from build123d import *

# Parameters (mm, degrees)
SKETCH1_W           = 150
SKETCH1_H           = 150
BOSS_EXTRUDE1_DEPTH = 3
SKETCH2_W           = 146
SKETCH2_H           = 146
BOSS_EXTRUDE2_DEPTH = 3
SKETCH3_W           = 142
SKETCH3_H           = 142
CUT_EXTRUDE1_DEPTH  = 3
EXTRUDE_THIN1_DEPTH = 3
CUT_EXTRUDE5_START  = -3
SKETCH5_W           = 71.2
SKETCH5_H           = 24.1
CUT_EXTRUDE5_DEPTH  = 3


with BuildPart() as part:
    # Sketch1 → Boss-Extrude1 (new body)
    with BuildSketch(Plane(origin=(0, 0, 0), x_dir=(1, 0, 0), z_dir=(0, 1, 0))):
        Rectangle(SKETCH1_W, SKETCH1_H)
    extrude(amount=-BOSS_EXTRUDE1_DEPTH)

    # Sketch2 → Boss-Extrude2 (add)
    with BuildSketch(Plane(origin=(0, 0, 0), x_dir=(1, 0, 0), z_dir=(0, 1, 0))):
        Rectangle(SKETCH2_W, SKETCH2_H)
    extrude(amount=BOSS_EXTRUDE2_DEPTH)

    # Sketch3 → Cut-Extrude1 (cut)
    with BuildSketch(Plane(origin=(0, 0, 0), x_dir=(1, 0, 0), z_dir=(0, 1, 0))):
        Rectangle(SKETCH3_W, SKETCH3_H)
    extrude(amount=CUT_EXTRUDE1_DEPTH, mode=Mode.SUBTRACT)

    # Sketch4 → Extrude-Thin1 (add)
    with BuildSketch(Plane(origin=(0, 0, 0), x_dir=(1, 0, 0), z_dir=(0, 1, 0))):
        Polygon((-71, 71), (71, -71), (70.292893219, -71.707106781), (-71.707106781, 70.292893219), align=None)
        Polygon((-71, -71), (71, 71), (71.707106781, 70.292893219), (-70.292893219, -71.707106781), align=None)
    extrude(amount=EXTRUDE_THIN1_DEPTH)

    # Sketch5 → Cut-Extrude5 (cut)
    with BuildSketch(Plane(origin=(0, 0, 0), x_dir=(1, 0, 0), z_dir=(0, 1, 0)).offset(CUT_EXTRUDE5_START)):
        with Locations((0, -52.95)):
            Rectangle(SKETCH5_W, SKETCH5_H)
    extrude(amount=CUT_EXTRUDE5_DEPTH, mode=Mode.SUBTRACT)


solid = part.part
Source: CAD feature listing. Evaluate the final solid. Frame: model axes, mm. Round coordinates to 2 decimals unless told otherwise and drop trailing zeros. Order: outer loops, then holes, each group sorted by start corner. A loop starts at its lowest first (then second) coordinate and runs counter-clockwise, first axis right, second up. Notation, with made-up numbers: (18.25, 59.5) -> (45.25, 59.5) arc R29 cw to (45.25, 84.5) -> close; hole circle Ø7 at (-38.75, 46). An arc over 180 degrees is marked (long way). Answer as CSV lines item,"result".
Item 1: Section A-A, the plane y = -1.3. Return loops of the section in (x, z), plus the area to 3 significant figures.
A:
outline,"(-75, -75) -> (75, -75) -> (75, 75) -> (-75, 75) -> close; hole (-35.6, 40.9) -> (35.6, 40.9) -> (35.6, 65) -> (-35.6, 65) -> close"
area,"20,800 mm²"
Item 2: Section B-B, the plane x = 28.5. Return loops of the section in (y, z).
A:
outline,"(-3, -75) -> (0, -75) -> (0, -73) -> (3, -73) -> (3, -71) -> (0, -71) -> (0, -28.5) -> (3, -28.5) -> (3, -27.09) -> (0, -27.09) -> (0, 28.5) -> (3, 28.5) -> (3, 29.91) -> (0, 29.91) -> (0, 40.9) -> (-3, 40.9) -> close; (-3, 65) -> (0, 65) -> (0, 71) -> (3, 71) -> (3, 73) -> (0, 73) -> (0, 75) -> (-3, 75) -> close"
Item 3: Section C-C, the plane x = 47. Return loops of the section in (y, z), plus the area to 3 significant figures.
A:
outline,"(-3, -75) -> (0, -75) -> (0, -73) -> (3, -73) -> (3, -71) -> (0, -71) -> (0, -47) -> (3, -47) -> (3, -45.59) -> (0, -45.59) -> (0, 47) -> (3, 47) -> (3, 48.41) -> (0, 48.41) -> (0, 71) -> (3, 71) -> (3, 73) -> (0, 73) -> (0, 75) -> (-3, 75) -> close"
area,"470 mm²"
Item 4: Line query: L1, parallel to X at y = 1.95, z = 7; L2, parallel to X at y = 1, z = 12.5; L3, parallel to Z at x = 66.5, y = 1.9. Output: solid intervals per line, ascending.
A:
L1,"-73 to -71, -7 to -5.59, 5.59 to 7, 71 to 73"
L2,"-73 to -71, -12.5 to -11.09, 11.09 to 12.5, 71 to 73"
L3,"-73 to -71, -66.5 to -65.09, 66.5 to 67.91, 71 to 73"
Item 5: Pin query (flat end, axial travel): pin 1 Ø0.9 at (x, y) = (4.5, 1.5) entering from -Z; pin 2 Ø0.9 at (x, y) = (19.5, 1) entering from +Z; pin 3 Ø3.5 at (y, z) = (2, -12) entering from +X. Return the tip coordinate at first contact, or that it passes through.
A:
pin 1,"z = -73"
pin 2,"z = 73"
pin 3,"x = 73"
Item 6: Pull-direction query (Z, two-part tool) for faces 1 (the face through (35, 1, -35)), 2 (the face through (-36, 1, -36)), 3 (the face through (-1, -3, -1)); classes: pulls with the +Z half, pulls with the -Z half, needs draft (parallel to the pull), parting line crosses it, or undercut.
A:
face 1,"undercut"
face 2,"undercut"
face 3,"needs draft"
Item 7: Section D-D, the plane z = -23. Return loops of the section in (x, y).
A:
outline,"(-75, -3) -> (75, -3) -> (75, 0) -> (73, 0) -> (73, 3) -> (71, 3) -> (71, 0) -> (24.41, 0) -> (24.41, 3) -> (23, 3) -> (23, 0) -> (-23, 0) -> (-23, 3) -> (-24.41, 3) -> (-24.41, 0) -> (-71, 0) -> (-71, 3) -> (-73, 3) -> (-73, 0) -> (-75, 0) -> close"
